Geometry check sheet. Reference: the model listing, model coordinates, mm. Face numbers are marked on the shaded views. A direction names the side the tool comes from. Round coordinates to 2 decimals unless told otherwise and drop trailing zeros. Loops run counter-clockwise (first coordinate to the right, second up) from the corner with the lowest first, then second, coordinate; pieces in that order, holes last. Notation, with made-up numbers: (81.5, -2) - (113.5, -2) arc R19 cw to (113.5, 11) - close; hole circle Ø4 at (78.25, 85). An arc over 180 degrees is marked (long way). Answer in a Markdown table with one row per item. Add a question column.
```python
from build123d import *

# Parameters (mm, degrees)
F1_DEPTH = 6.35
F2_SIZE  = 1.5748


with BuildPart() as f1:
    # F0 (on Top) → F1 (new body)
    with BuildSketch(Plane.XY):
        Polygon((9.525, 35.814), (0, 35.814), (0, 0), (35.814, 0), (35.814, 9.525), align=None)
        with BuildLine():
            Line((6.35, 7.9248), (6.35, 26.20684))
            ThreePointArc((6.35, 26.20684), (7.32215, 27.661766), (9.038352, 27.320392))
            Line((9.038352, 27.320392), (27.320392, 9.038352))
            ThreePointArc((27.320392, 9.038352), (27.661766, 7.32215), (26.20684, 6.35))
            Line((26.20684, 6.35), (7.9248, 6.35))
            ThreePointArc((7.9248, 6.35), (6.811248, 6.811248), (6.35, 7.9248))
        make_face(mode=Mode.SUBTRACT)
    extrude(amount=F1_DEPTH)

    # F2
    f2_edges = [f1.edges().sort_by_distance(p)[0] for p in [
        (0, 0, 3.175),
    ]]
    chamfer(f2_edges, length=F2_SIZE)


solid = f1.part
```
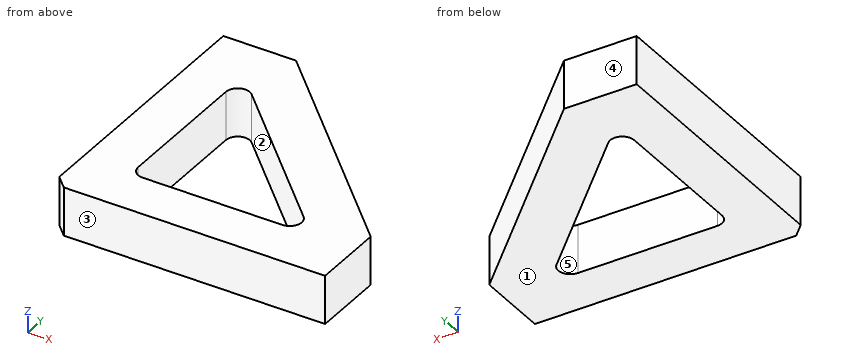
Q1. Cross-section at A-A, the plane z = 2.5. Enter the section's corners in (x, y) (3 decimals).
Q2. Release check for a two-part mould opening along Y. For the marked faces 3, 4 and 5 record: +Y half, -Y half, draft (parallel to the pull), parting line (faces both ways), or undercut.
Q3. Scan lines: line 1 (Y direction, x = 12, z = 4.25); line 2 (Y direction, x = 10.5, z = 3); line 3 (X direction, y = 23, z = 4.25). Record each from-to range of solid material in increasing order. Write a range as from..to.
Q4. Cross-section at B-B, the plane y = 14. Enter the section's corners in (x, z).
Q5. Cross-section at C-C, the plane x = 25.5. Enter the section's corners in (y, z).
Q6. Set-up check for the marked faces 1 and 2: record each of +Z, -Z, +X, -X, +Y, -Y from which the full face is reachable in a straight line by a thin tool's end or side.
Q7. Depth check by flat-ended pin: P1, Ø1.9, axis at y = 13.5, z = 2.5, coming from the +X side; P2, Ø3, axis at x = 15.5, z = 2, coming from the +Y side; P3, Ø2, axis at x = 28.5, y = 10.5, coming from the -Z side; P4, Ø1, axis at y = 25, z = 4.5, coming from the +X side. Enter the tip coordinate at first touch or a pass-through.
Q8. Cross-section at D-D, the plane y = 28.5. Enter the section's corners in (x, z), plus the area to 3 significant figures.
Check sheet entries:
| question | item | result |
|---|---|---|
| 1 | outline | (0, 1.575) - (1.575, 0) - (35.814, 0) - (35.814, 9.525) - (9.525, 35.814) - (0, 35.814) - close; hole (6.35, 7.925) arc R1.575 ccw to (7.925, 6.35) - (26.207, 6.35) arc R1.575 ccw to (27.32, 9.038) - (9.038, 27.32) arc R1.575 ccw to (6.35, 26.207) - close |
| 2 | face 3 | -Y half |
| 2 | face 4 | +Y half |
| 2 | face 5 | undercut |
| 3 | line 1 | 0..6.35, 24.36..33.34 |
| 3 | line 2 | 0..6.35, 25.86..34.84 |
| 3 | line 3 | 0..6.35, 13.36..22.34 |
| 4 | outline | (0, 0) - (6.35, 0) - (6.35, 6.35) - (0, 6.35) - close; (22.36, 0) - (31.34, 0) - (31.34, 6.35) - (22.36, 6.35) - close |
| 5 | outline | (0, 0) - (6.35, 0) - (6.35, 6.35) - (0, 6.35) - close; (10.86, 0) - (19.84, 0) - (19.84, 6.35) - (10.86, 6.35) - close |
| 6 | face 1 | -Z, +X, -X, +Y, -Y |
| 6 | face 2 | +Z, -Z |
| 7 | P1 | x = 32.79 |
| 7 | P2 | y = 31.34 |
| 7 | P3 | z = 0 |
| 7 | P4 | x = 20.84 |
| 8 | outline | (0, 0) - (16.84, 0) - (16.84, 6.35) - (0, 6.35) - close |
| 8 | area | 107 mm² |
